from build123d import *

# Parameters (mm, degrees)
F0_W     = 73.66
F0_H     = 97.79
F1_DEPTH = 9.525


# Not quite as in the source:
# - a length typed as a fraction of an inch, garbled in the dataset ("3 / 203.2 mm" for 3/8 in), is restored


with BuildPart() as f1:
    # F0 (on Top) → F1 (new body)
    with BuildSketch(Plane.XY):
        Rectangle(F0_W, F0_H)
    extrude(amount=F1_DEPTH)

    # F2 (on Right) → F3 (revolve)
    with BuildSketch(Plane.YZ):
        Polygon((35.179, 0), (33.401, 0), (33.401, -5.334), (37.5285, -5.334), (37.5285, -1.524), (35.179, -1.524), align=None)
    revolve(axis=Axis((0, 33.401, -2.667), (0, 0, -1)))

    # F2 (on Right) → F4 (revolve)
    with BuildSketch(Plane.YZ):
        Polygon((-33.401, 0), (-35.179, 0), (-35.179, -1.524), (-37.5285, -1.524), (-37.5285, -5.334), (-33.401, -5.334), align=None)
    revolve(axis=Axis((0, -33.401, -2.667), (0, 0, -1)))


solid = f1.part
Could you check a few things on this model? Use its own coordinates, in mm. A direction names the side the tool comes from. Round coordinates to 2 decimals unless told otherwise and drop trailing zeros. Order: outer loops, then holes, each group sorted by start corner. A loop starts at its lowest first (then second) coordinate and runs counter-clockwise, first axis right, second up.
(1) I'm going to push flat-ended pins straight in: pin 1 (4 mm diameter, centred on x = 28, y = 2, fed in from -Z); pin 2 (8 mm diameter, centred on x = -29.5, z = -3.5, fed in from -Y) (3 decimals). Where does each tip first touch, or does it pass through?
Response values:
pin 1: stops at z = 0
pin 2: stops at y = -48.895
(2) Which directions (+Z, -Z, +X, -X, +Y, -Y) give clear straight access to the entire face, cutting with the end or side of a thin tool? Please do faces 4 (the cylindrical face through (0.181, 29.277, -3.402)), 5 (the cylindrical face through (0.53, 35.1, -0.75)), 6 (the flat face through (0, 33, -5.334)).
Response values:
face 4: -Z
face 5: none
face 6: -Z, +X, -X, +Y, -Y
(3) Imagine slicing it at B-B (y = 33). Write out the boundary of the cut face in (x, z) (3 decimals), plus the area to 3 significant figures.
Response values:
outline: (-36.83, 0) - (-1.732, 0) - (-1.732, -1.524) - (-4.108, -1.524) - (-4.108, -5.334) - (4.108, -5.334) - (4.108, -1.524) - (1.732, -1.524) - (1.732, 0) - (36.83, 0) - (36.83, 9.525) - (-36.83, 9.525) - close
area: 738 mm2
(4) Imagine slicing it at C-C (z = -4). Write out the boundary of the cut face in (x, y) (1 decimal), plus the area to 3 significant figures.
Response values:
outline: circle Ø8.3 at (0, -33.4); circle Ø8.3 at (0, 33.4)
area: 107 mm2
(5) Imagine slicing it at A-A (x = 0). Write out the boundary of the cut face in (y, z) (1 decimal), plus the area to 3 significant figures.
Response values:
outline: (-48.9, 0) - (-35.2, 0) - (-35.2, -1.5) - (-37.5, -1.5) - (-37.5, -5.3) - (-29.3, -5.3) - (-29.3, -1.5) - (-31.6, -1.5) - (-31.6, 0) - (31.6, 0) - (31.6, -1.5) - (29.3, -1.5) - (29.3, -5.3) - (37.5, -5.3) - (37.5, -1.5) - (35.2, -1.5) - (35.2, 0) - (48.9, 0) - (48.9, 9.5) - (-48.9, 9.5) - close
area: 1,010 mm2
(6) Please list where these lines run through material, in increasing order: line 1 along Z through (x, y) = (-15, 9) (3 decimals); line 2 along Y through (x, z) = (0.5, -1.25); line 3 along Y through (x, z) = (2, -3.5).
Response values:
line 1: z = 0 to 9.525
line 2: y = -35.11 to -31.69, 31.69 to 35.11
line 3: y = -37.01 to -29.79, 29.79 to 37.01
(7) Imagine slicing it at D-D (x = -10). Write out the boundary of the cut face in (y, z) (3 decimals), plus the area to 3 significant figures.
Response values:
outline: (-48.895, 0) - (48.895, 0) - (48.895, 9.525) - (-48.895, 9.525) - close
area: 931 mm2
(8) If we mould it in two halves opening along Z, with no side actions, what happens to faces 1 (the flat face through (-0.9, 35.2, -1.524)), 2 (the flat face through (-1, 48.895, 5)), 3 (the flat face through (-1, 1, 9.525))? For each: released by +Z, released by -Z, zero draft, split by the parting line, or undercut.
Response values:
face 1: undercut
face 2: zero draft
face 3: released by +Z
